```python
from build123d import *

# Parameters (mm, degrees)
F1_DEPTH = 7
F2_SIZE  = 3.175
F3_DEPTH = 7.001


with BuildPart() as f1:
    # F0 (on Top) → F1 (new body)
    with BuildSketch(Plane.XY):
        with BuildLine():
            Line((13.6507254272, 7.88125), (0, 42.5250102))
            Line((0, 42.5250102), (0, 15.7625))
            ThreePointArc((0, 15.7625), (7.88125, 13.6507254272), (13.6507254272, 7.88125))
        make_face()
        with BuildLine():
            Line((0, 15.7625), (0, 42.5250102))
            Line((0, 42.5250102), (-13.6507254272, 7.88125))
            ThreePointArc((-13.6507254272, 7.88125), (-7.88125, 13.6507254272), (0, 15.7625))
        make_face()
        with BuildLine():
            ThreePointArc((-13.6507254272, -7.88125), (-15.7625, 0), (-13.6507254272, 7.88125))
            Line((-13.6507254272, 7.88125), (-36.8277391294, -21.2625051))
            Line((-36.8277391294, -21.2625051), (-13.6507254272, -7.88125))
        make_face()
        with BuildLine():
            Line((-36.8277391294, -21.2625051), (0, -15.7625))
            ThreePointArc((0, -15.7625), (-7.88125, -13.6507254272), (-13.6507254272, -7.88125))
            Line((-13.6507254272, -7.88125), (-36.8277391294, -21.2625051))
        make_face()
        with BuildLine():
            Line((0, -15.7625), (36.8277391294, -21.2625051))
            Line((36.8277391294, -21.2625051), (13.6507254272, -7.88125))
            ThreePointArc((13.6507254272, -7.88125), (7.88125, -13.6507254272), (0, -15.7625))
        make_face()
        with BuildLine():
            Line((13.6507254272, -7.88125), (36.8277391294, -21.2625051))
            Line((36.8277391294, -21.2625051), (13.6507254272, 7.88125))
            ThreePointArc((13.6507254272, 7.88125), (15.2254058369, 4.0796351984), (15.7625, 0))
            ThreePointArc((15.7625, 0), (15.2254058369, -4.0796351984), (13.6507254272, -7.88125))
        make_face()
        with BuildLine():
            Line((0, 11), (0, 15.7625))
            ThreePointArc((0, 15.7625), (-7.88125, 13.6507254272), (-13.6507254272, 7.88125))
            Line((-13.6507254272, 7.88125), (-9.5262794416, 5.5))
            ThreePointArc((-9.5262794416, 5.5), (-5.5, 9.5262794416), (0, 11))
        make_face()
        with BuildLine():
            Line((9.5262794416, 5.5), (13.6507254272, 7.88125))
            ThreePointArc((13.6507254272, 7.88125), (7.88125, 13.6507254272), (0, 15.7625))
            Line((0, 15.7625), (0, 11))
            ThreePointArc((0, 11), (5.5, 9.5262794416), (9.5262794416, 5.5))
        make_face()
        with BuildLine():
            ThreePointArc((15.7625, 0), (15.2254058369, 4.0796351984), (13.6507254272, 7.88125))
            Line((13.6507254272, 7.88125), (9.5262794416, 5.5))
            ThreePointArc((9.5262794416, 5.5), (10.6251840892, 2.8470094961), (11, 0))
            ThreePointArc((11, 0), (10.6251840892, -2.8470094961), (9.5262794416, -5.5))
            Line((9.5262794416, -5.5), (13.6507254272, -7.88125))
            ThreePointArc((13.6507254272, -7.88125), (15.2254058369, -4.0796351984), (15.7625, 0))
        make_face()
        with BuildLine():
            ThreePointArc((0, -15.7625), (7.88125, -13.6507254272), (13.6507254272, -7.88125))
            Line((13.6507254272, -7.88125), (9.5262794416, -5.5))
            ThreePointArc((9.5262794416, -5.5), (5.5, -9.5262794416), (0, -11))
            Line((0, -11), (0, -15.7625))
        make_face()
        with BuildLine():
            ThreePointArc((-13.6507254272, -7.88125), (-7.88125, -13.6507254272), (0, -15.7625))
            Line((0, -15.7625), (0, -11))
            ThreePointArc((0, -11), (-5.5, -9.5262794416), (-9.5262794416, -5.5))
            Line((-9.5262794416, -5.5), (-13.6507254272, -7.88125))
        make_face()
        with BuildLine():
            Line((-9.5262794416, 5.5), (-13.6507254272, 7.88125))
            ThreePointArc((-13.6507254272, 7.88125), (-15.7625, 0), (-13.6507254272, -7.88125))
            Line((-13.6507254272, -7.88125), (-9.5262794416, -5.5))
            ThreePointArc((-9.5262794416, -5.5), (-11, 0), (-9.5262794416, 5.5))
        make_face()
        with BuildLine():
            Line((0, 0), (-9.5262794416, 5.5))
            ThreePointArc((-9.5262794416, 5.5), (-11, 0), (-9.5262794416, -5.5))
            Line((-9.5262794416, -5.5), (0, 0))
        make_face()
        with BuildLine():
            ThreePointArc((-9.5262794416, -5.5), (-5.5, -9.5262794416), (0, -11))
            Line((0, -11), (0, 0))
            Line((0, 0), (-9.5262794416, -5.5))
        make_face()
        with BuildLine():
            ThreePointArc((0, -11), (5.5, -9.5262794416), (9.5262794416, -5.5))
            Line((9.5262794416, -5.5), (0, 0))
            Line((0, 0), (0, -11))
        make_face()
        with BuildLine():
            ThreePointArc((11, 0), (10.6251840892, 2.8470094961), (9.5262794416, 5.5))
            Line((9.5262794416, 5.5), (0, 0))
            Line((0, 0), (9.5262794416, -5.5))
            ThreePointArc((9.5262794416, -5.5), (10.6251840892, -2.8470094961), (11, 0))
        make_face()
        with BuildLine():
            Line((0, 0), (9.5262794416, 5.5))
            ThreePointArc((9.5262794416, 5.5), (5.5, 9.5262794416), (0, 11))
            Line((0, 11), (0, 0))
        make_face()
        with BuildLine():
            Line((0, 0), (0, 11))
            ThreePointArc((0, 11), (-5.5, 9.5262794416), (-9.5262794416, 5.5))
            Line((-9.5262794416, 5.5), (0, 0))
        make_face()
    extrude(amount=F1_DEPTH)

    # F2
    f2_edges = [f1.edges().sort_by_distance(p)[0] for p in [
        (-18.41387, -18.512503, 7),
        (-6.825363, 25.20313, 7),
        (-25.239232, -6.690628, 7),
        (18.41387, -18.512503, 7),
        (25.239232, -6.690628, 7),
        (6.825363, 25.20313, 7),
        (-6.825363, 25.20313, 0),
        (-25.239232, -6.690628, 0),
        (-18.41387, -18.512503, 0),
        (18.41387, -18.512503, 0),
        (25.239232, -6.690628, 0),
        (6.825363, 25.20313, 0),
    ]]
    chamfer(f2_edges, length=F2_SIZE)

    # F0 (on Top) → F3 (cut, through all)
    with BuildSketch(Plane.XY):
        with BuildLine():
            ThreePointArc((0, -11), (5.5, -9.5262794416), (9.5262794416, -5.5))
            Line((9.5262794416, -5.5), (0, 0))
            Line((0, 0), (0, -11))
        make_face()
        with BuildLine():
            ThreePointArc((-9.5262794416, -5.5), (-5.5, -9.5262794416), (0, -11))
            Line((0, -11), (0, 0))
            Line((0, 0), (-9.5262794416, -5.5))
        make_face()
        with BuildLine():
            Line((0, 0), (-9.5262794416, 5.5))
            ThreePointArc((-9.5262794416, 5.5), (-11, 0), (-9.5262794416, -5.5))
            Line((-9.5262794416, -5.5), (0, 0))
        make_face()
        with BuildLine():
            Line((0, 0), (0, 11))
            ThreePointArc((0, 11), (-5.5, 9.5262794416), (-9.5262794416, 5.5))
            Line((-9.5262794416, 5.5), (0, 0))
        make_face()
        with BuildLine():
            Line((0, 0), (9.5262794416, 5.5))
            ThreePointArc((9.5262794416, 5.5), (5.5, 9.5262794416), (0, 11))
            Line((0, 11), (0, 0))
        make_face()
        with BuildLine():
            ThreePointArc((11, 0), (10.6251840892, 2.8470094961), (9.5262794416, 5.5))
            Line((9.5262794416, 5.5), (0, 0))
            Line((0, 0), (9.5262794416, -5.5))
            ThreePointArc((9.5262794416, -5.5), (10.6251840892, -2.8470094961), (11, 0))
        make_face()
    extrude(amount=F3_DEPTH, mode=Mode.SUBTRACT)


solid = f1.part
```
The listing builds one solid part. Answer for the finished solid, in the listing's coordinates (mm). A direction names the side the tool comes from. Give positions to 0.01 mm unless a question says otherwise; leave off trailing zeros. Order: outer loops, then holes, each group sorted by start corner. A loop starts at its lowest first (then second) coordinate and runs counter-clockwise, first axis right, second up. Notation, with made-up numbers: (13.25, 37) -> (44.25, 37) arc R12 cw to (44.25, 59) -> close; hole circle Ø11 at (85, -29.5). An arc over 180 degrees is marked (long way). One line per item, written item: value.
1) Find section A-A, the plane z = 6. Determine the outline of the cut face in (x, y), plus the area to 3 significant figures.
Reported:
outline: (-31.69, -18.3) -> (0, -13.56) -> (31.69, -18.3) -> (11.75, 6.78) -> (0, 36.59) -> (-11.75, 6.78) -> close; hole circle Ø22 at (0, 0)
area: 909 mm^2
2) Find section C-C, the plane x = -17.5. Determine the outline of the cut face in (y, z) (3 decimals).
Reported:
outline: (-18.376, 3.175) -> (-15.166, 0) -> (-2.06, 0) -> (3.041, 3.175) -> (3.041, 3.825) -> (-2.06, 7) -> (-15.166, 7) -> (-18.376, 3.825) -> close
3) Flat-ended cylindrical pins translate along their axes: P1, Ø1, axis at y = 20.5, z = 2.5, coming from the -X side; P2, Ø3, axis at x = -0.5, z = 1, coming from the -Y side; P3, Ø1, axis at x = 26, z = 6, coming from the -Y side. Find the tip coordinate at first contact, or state that the pin passes through.
Reported:
P1: stops at x = -8.53
P2: stops at y = -15.17
P3: stops at y = -17.96
4) Find section D-D, the plane y = 23. Determine the outline of the cut face in (x, z) (3 decimals).
Reported:
outline: (-7.693, 3.175) -> (-4.281, 0) -> (4.281, 0) -> (7.693, 3.175) -> (7.693, 3.825) -> (4.281, 7) -> (-4.281, 7) -> (-7.693, 3.825) -> close
5) Determine the mould class of faces 5 (the flat face through (-5.32, 24.64, 5.43)), 6 (the flat face through (5.511, 24.147, 1.565)), 7 (the flat face through (18.16, -16.85, 5.43)) for opening direction X: pulls with the +X half, pulls with the -X half, needs draft (parallel to the pull), parting line crosses it, or undercut.
Reported:
face 5: pulls with the -X half
face 6: pulls with the +X half
face 7: undercut
6) Find the intervals of material crossed by line 1 (X direction, y = 4, z = 1.5); line 2 (X direction, y = -6, z = 0.5); line 3 (Y direction, x = -30, z = 3.75), in increasing order.
Reported:
line 1: x = -14.6 to -10.25, 10.25 to 14.6
line 2: x = -21.27 to -9.22, 9.22 to 21.27
line 3: y = -20.24 to -12.68
7) Find section B-B, the plane y = -6.5. Determine the outline of the cut face in (x, z) (3 decimals), plus the area to 3 significant figures.
Reported:
outline: (-25.088, 3.175) -> (-21.031, 0) -> (-8.874, 0) -> (-8.874, 7) -> (-21.031, 7) -> (-25.088, 3.825) -> close; (8.874, 0) -> (21.031, 0) -> (25.088, 3.175) -> (25.088, 3.825) -> (21.031, 7) -> (8.874, 7) -> close
area: 201 mm^2
8) A tool of negligible diameter and unlimited length cuts with its end or side. For faces 1 (the flat face through (-18.67, -18.55, 3.5)), 2 (the flat face through (18.16, -16.85, 1.57)), 3 (the flat face through (24, -7.71, 1.57)), 4 (the flat face through (-18.678, -16.924, 5.435)), from which of +Z, -Z, +X, -X, +Y, -Y can it reach the whole face along a straight path? Write none if from no direction.
Reported:
face 1: +Z, -Z, -Y
face 2: -Z, -Y
face 3: -Z, +X, +Y
face 4: +Z, -Y
